```python
from build123d import *

# Parameters (mm, degrees)
F0_W   = 20
F0_H   = 5
F0_W_2 = 50
F0_H_2 = 10
F0_W_3 = 230


with BuildPart() as f1:
    # F0 (on Top) → F1 (revolve)
    with BuildSketch(Plane.XY):
        with Locations((-60, 2.5)):
            Rectangle(F0_W, F0_H)
        with Locations((-25, 10)):
            Rectangle(F0_W_2, F0_H_2)
        with Locations((-25, 2.5)):
            Rectangle(F0_W_2, F0_H)
        with Locations((115, 2.5)):
            Rectangle(F0_W_3, F0_H)
    revolve(axis=Axis((80, 0, 0), (1, 0, 0)))


solid = f1.part
```
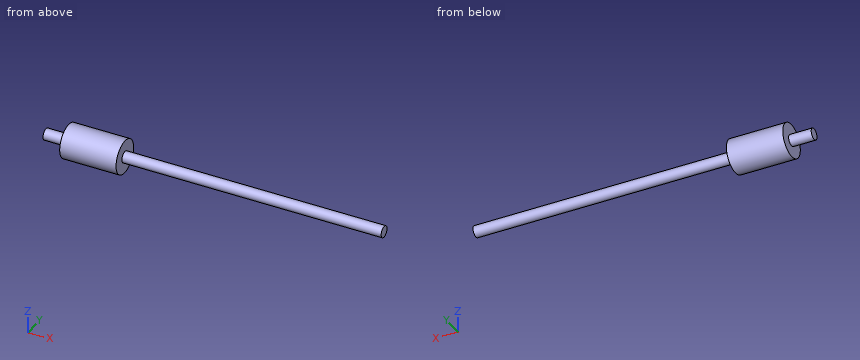
The listing builds one solid part. Answer for the finished solid, in the listing's coordinates (mm). Round coordinates to 2 decimals unless told otherwise and drop trailing zeros. Write each loop counter-clockwise with the first axis right and the second up, starting at its lowest first coordinate (ties: lowest second). Pieces come first, ordered by that corner, then holes. Notation, with made-up numbers: (80.5, 85) -> (107.5, 85) arc R18 ccw to (107.5, 112) -> close; hole circle Ø11 at (19, 13). An arc over 180 degrees is marked (long way). Answer as a JSON object with one key per item and string values. Group by question number.
Q1. Section A-A (y = 0) is taken. Write down the section's boundary in (x, z), plus the area to 3 significant figures.
Q2. Straight lines are drawn through the part: line 1 along X through (y, z) = (-10.5, 5.5); line 2 along Y through (x, z) = (-47.5, 2.25); line 3 along Y through (x, z) = (199, 0.25). For each, find the intervals that lie inside material, in ascending order.
Q3. Section C-C (x = 149.5) is taken. Write down the section's boundary in (y, z), plus the area to 3 significant figures.
Q4. Each of these flat-tipped pins is pushed along its axis until it touches: pin 1 Ø8 at (x, y) = (75.5, 11) entering from -Z; pin 2 Ø6 at (x, y) = (13.5, -7) entering from -Z; pin 3 Ø2 at (y, z) = (7, -8.5) entering from +X; pin 4 Ø5 at (x, y) = (-15.5, -3) entering from -Z. Where does it stop, or does it pass through?
Check values:
{
 "1": {"outline": "(-70, -5) -> (-50, -5) -> (-50, -15) -> (0, -15) -> (0, -5) -> (230, -5) -> (230, 5) -> (0, 5) -> (0, 15) -> (-50, 15) -> (-50, 5) -> (-70, 5) -> close", "area": "4,000 mm^2"},
 "2": {"line 1": "-50 to 0", "line 2": "-14.83 to 14.83", "line 3": "-4.99 to 4.99"},
 "3": {"outline": "circle Ø10 at (0, 0)", "area": "78.5 mm^2"},
 "4": {"pin 1": "through", "pin 2": "z = -3", "pin 3": "x = 0", "pin 4": "z = -14.99"}
}
